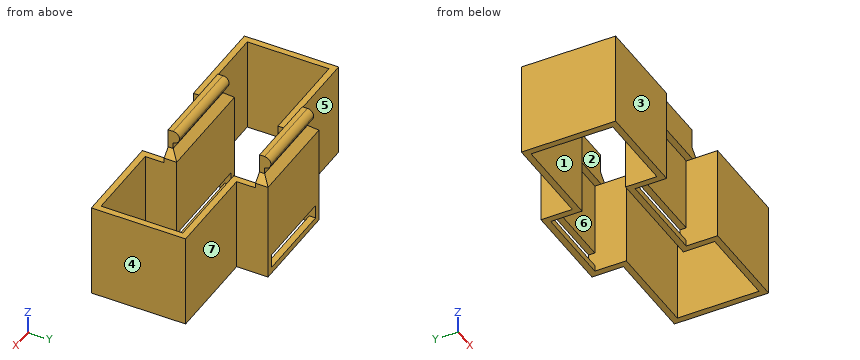
```python
from build123d import *

# Parameters (mm, degrees)
F3_DEPTH  = 15
F4_W      = 1
F4_H      = 1
F4_W_2    = 15
F4_W_3    = 13
F5_DEPTH  = 2
F6_SIZE   = 1.2
F7_DEPTH  = 3
F8_W      = 14.6
F8_H      = 2
F9_W      = 12.6
F9_H      = 2
F10_DEPTH = 1
F11_R     = 0.99999
F12_W     = 15
F12_H     = 2.2
F13_W     = 13
F13_H     = 2.2
F14_DEPTH = 1


# Not quite as in the source:
# - a fillet or chamfer is up to 0.001 mm smaller than in the source, because OpenCascade refuses the exact size


with BuildPart() as f3:
    # F2 (on Top) → F3 (new body)
    with BuildSketch(Plane.XY):
        Polygon((-39.3307432532, 0), (-24.3307432532, 0), (-24.3307432532, 5), (-24.3307432532, 6), (-25.3307432532, 6), (-25.3307432532, 1), (-38.3307432532, 1), (-38.3307432532, 14), (-25.3307432532, 14), (-24.3307432532, 14), (-24.3307432532, 15), (-39.3307432532, 15), align=None)
        Polygon((-24.3307432532, 6), (-24.3307432532, 5), (-9.3307432532, 5), (-9.3307432532, 6), (-10.3307432532, 6), (-23.3307432532, 6), align=None)
        Polygon((-9.3307432532, 6), (-9.3307432532, 5), (-9.3307432532, 0), (5.6692567468, 0), (5.6692567468, 15), (-9.3307432532, 15), (-9.3307432532, 14), (-8.3307432532, 14), (4.6692567468, 14), (4.6692567468, 1), (-8.3307432532, 1), (-8.3307432532, 6), align=None)
        Polygon((-24.3307432532, 20), (-24.3307432532, 15), (-24.3307432532, 14), (-23.3307432532, 14), (-23.3307432532, 19), (-10.3307432532, 19), (-10.3307432532, 14), (-9.3307432532, 14), (-9.3307432532, 15), (-9.3307432532, 20), align=None)
    extrude(amount=F3_DEPTH)

    # F4 (on face) → F5 (join)
    with BuildSketch(Plane.XY.offset(15)):
        Polygon((-8.3307432532, 6), (-25.3307432532, 6), (-25.3307432532, 5), (-24.3307432532, 5), (-9.3307432532, 5), (-8.3307432532, 5), align=None)
        with Locations((-8.8307432532, 4.5)):
            Rectangle(F4_W, F4_H)
        with Locations((-16.8307432532, 4.5)):
            Rectangle(F4_W_2, F4_H)
        with Locations((-24.8307432532, 4.5)):
            Rectangle(F4_W, F4_H)
        Polygon((-24.3307432532, 19), (-23.3307432532, 19), (-10.3307432532, 19), (-9.3307432532, 19), (-9.3307432532, 20), (-24.3307432532, 20), align=None)
        with Locations((-23.8307432532, 18.5)):
            Rectangle(F4_W, F4_H)
        with Locations((-16.8307432532, 18.5)):
            Rectangle(F4_W_3, F4_H)
        with Locations((-9.8307432532, 18.5)):
            Rectangle(F4_W, F4_H)
    extrude(amount=F5_DEPTH)

    # F6
    f6_edges = [f3.edges().sort_by_distance(p)[0] for p in [
        (-16.830743, 6, 17),
        (-25.330743, 5, 17),
        (-8.330743, 5, 17),
        (-16.830743, 20, 17),
        (-24.330743, 19, 17),
        (-9.330743, 19, 17),
    ]]
    chamfer(f6_edges, length=F6_SIZE)

    # F7 (add): faces of the model
    f7_faces = [f3.faces().sort_by_distance(p)[0] for p in [
        (-16.8307432532, 4.4, 17),
        (-16.8307432532, 18.4, 17),
    ]]
    extrude(f7_faces, amount=F7_DEPTH)

    # F8 (on face) + F9 (on face) → F10 (join)
    with BuildSketch(Plane(origin=(0, 4.8, 0), x_dir=(-1, 0, 0), z_dir=(0, 1, 0))):
        with Locations((16.8307432532, 19)):
            Rectangle(F8_W, F8_H)
    with BuildSketch(Plane(origin=(0, 18.8, 0), x_dir=(-1, 0, 0), z_dir=(0, 1, 0))):
        with Locations((16.8307432532, 19)):
            Rectangle(F9_W, F9_H)
    extrude(amount=F10_DEPTH)

    # F11 (radius 1 in the source; OpenCascade refuses exactly that, so slightly less here)
    f11_edges = [f3.edges().sort_by_distance(p)[0] for p in [
        (-16.830743, 5.8, 20),
        (-16.830743, 5.8, 18),
        (-16.830743, 19.8, 20),
        (-16.830743, 19.8, 18),
    ]]
    fillet(f11_edges, radius=F11_R)

    # F12 (on face) + F13 (on face) → F14 (cut, through all)
    with BuildSketch(Plane.XZ.offset(-5)):
        with Locations((-16.8307432532, 2.1)):
            Rectangle(F12_W, F12_H)
    with BuildSketch(Plane.XZ.offset(-19)):
        with Locations((-16.8307432532, 2.1)):
            Rectangle(F13_W, F13_H)
    extrude(amount=-F14_DEPTH, mode=Mode.SUBTRACT)


solid = f3.part
```
Check sheet for the modelled part. Datum: model origin and axes. Units: mm. Face numbers are marked on the shaded views. A direction names the side the tool comes from. Give positions to 0.01 mm unless a question says otherwise; leave off trailing zeros. Write each loop counter-clockwise with the first axis right and the second up, starting at its lowest first coordinate (ties: lowest second). Pieces come first, ordered by that corner, then holes. Notation, with made-up numbers: (-34.75, -36.5) - (4.25, -36.5) arc R10 cw to (4.25, -23.5) - close; hole circle Ø9 at (-38, -18.75). An arc over 180 degrees is marked (long way). Answer as a JSON object with one key per item and string values. Group by question number.
1) Sectioned sample at B-B (x = -12). Give the number of separate pieces and of enclosed holes in the cut face, then the cut area to 3 significant figures.
2) Access from +Z, -Z, +X, -X, +Y, -Y to the whole of each face (thin tool, end or side, straight path). Record for the marked faces 5, 6 and 7.
3) Sectioned sample at D-D (x = -31). Record the cut outline in (y, z).
4) Release check for a two-part mould opening along Y. For the marked faces 1, 2, 3 and 4 record: pulls with the +Y half, pulls with the -Y half, needs draft (parallel to the pull), parting line crosses it, or undercut.
5) Depth check by flat-ended pin: P1, Ø10.5, axis at x = -0.5, z = 7.5, coming from the +Y side; P2, Ø2.5, axis at y = 18, z = 9.5, coming from the +X side; P3, Ø6, axis at x = -28, y = 12, coming from the +Z side. Enter the tip coordinate at first touch or a pass-through.
6) Thickness scan on probe 1 along X at (y, z) = (2, 11); probe 2 along X at (y, z) = (18.5, 12); probe 3 along Y at (x, z) = (-35, 3.75). Record the ranges inside material, lowest first. Write a range as from..to.
7) Sectioned sample at A-A (z = 1.5). Record the cut outline in (x, y).
8) Sectioned sample at C-C (y = 17.25). Record the cut outline in (x, z), then the cut area to 3 significant figures.
Geometry results:
{
 "1": {"separate pieces": "4", "enclosed holes": "0", "area": "40.1 mm^2"},
 "2": {"face 5": "+Z, -Z, -X, +Y", "face 6": "-Z", "face 7": "+Z, -Z, +X, +Y"},
 "3": {"outline": "(0, 0) - (1, 0) - (1, 15) - (0, 15) - close; (14, 0) - (15, 0) - (15, 15) - (14, 15) - close"},
 "4": {"face 1": "undercut", "face 2": "undercut", "face 3": "pulls with the -Y half", "face 4": "needs draft"},
 "5": {"P1": "stops at y = 15", "P2": "stops at x = -9.33", "P3": "stops at z = 15"},
 "6": {"probe 1": "x = -39.33..-38.33, -25.33..-24.33, -9.33..-8.33, 4.67..5.67", "probe 2": "x = -24.33..-23.33, -10.33..-9.33", "probe 3": "y = 0..1, 14..15"},
 "7": {"outline": "(-39.33, 0) - (-24.33, 0) - (-24.33, 6) - (-25.33, 6) - (-25.33, 1) - (-38.33, 1) - (-38.33, 14) - (-23.33, 14) - (-23.33, 20) - (-24.33, 20) - (-24.33, 15) - (-39.33, 15) - close; (-10.33, 14) - (4.67, 14) - (4.67, 1) - (-8.33, 1) - (-8.33, 6) - (-9.33, 6) - (-9.33, 0) - (5.67, 0) - (5.67, 15) - (-9.33, 15) - (-9.33, 20) - (-10.33, 20) - close"},
 "8": {"outline": "(-24.33, 0) - (-23.33, 0) - (-23.33, 15) - (-24.33, 15) - close; (-10.33, 0) - (-9.33, 0) - (-9.33, 15) - (-10.33, 15) - close", "area": "30.0 mm^2"}
}
